Input: part model. Units: mm. Frame: model coordinates. A direction names the side the tool comes from. Coordinates: 2 decimals unless noted, no trailing zeros. Write each loop counter-clockwise with the first axis right and the second up, starting at its lowest first coordinate (ties: lowest second). Pieces come first, ordered by that corner, then holes. Notation, with made-up numbers: M 42.25,15.25 L 49.25,15.25 A34 ccw 49.25,49.25 Z; hole C 50,-24.75 d6. An arc over 180 degrees is marked long. Use one line per item in the form item = value.
Autodesk Inventor part; units mm, degrees
ref_plane "YZ Plane" through (0, 0, 0) normal (1, 0, 0) x (0, 1, 0)
ref_plane "XZ Plane" through (0, 0, 0) normal (0, 1, 0) x (-1, 0, 0)
ref_plane "XY Plane" through (0, 0, 0) normal (0, 0, 1) x (1, 0, 0)
sketch "스케치1" plane through (0, 0, 0) normal (0, 0, 1) x (1, 0, 0)
  line L0 (0, 0) -> (28, 0)
  line L1 (28, 0) -> (28, 33)
  line L2 (28, 33) -> (0, 33)
  line L3 (0, 33) -> (0, 0)
  line L4 (0, 34) -> (28, 34)
  line L5 (28, 34) -> (28, -1)
  line L6 (28, -1) -> (0, -1)
  line L7 (0, -1) -> (0, 34)
  circle A0 centre (-3.95, 14.85) radius 1.65
  circle A1 centre (31.95, 14.85) radius 1.65
  circle A2 centre (14, 14.85) radius 22.1
  line L8 (0, 34) -> (-8.1, 14.85)
  line L9 (-8.1, 14.85) -> (0, -1)
  line L10 (28, -1) -> (36.1, 14.85)
  line L11 (36.1, 14.85) -> (28, 34)
  point P0 (29.3923, 30.7084)
  point P1 (26.609, 33)
  point P2 (1.391, 33)
  point P3 (-1.3923, 30.7084)
  point P4 (0, 31.95)
  point P5 (28, 31.95)
  dimension "d0" = 28
  dimension "d1" = 33
  dimension "d2" = 28
  dimension "d3" = 35
  dimension "d4" = 1
  dimension "d5" = 3.3
  dimension "d6" = 3.3
  dimension "d7" = 35.9
  dimension "d8" = 3.95
  dimension "d9" = 15.85
  dimension "d10" = 44.2
extrude "돌출1" add sketch "스케치1" against normal blind 3.9 contours L3 A2 L2 L1 L0 | L7 L9 L8 A2 L3 | L0 L5 L6 L7 | L1 A2 L11 L10 L5 | A2 L8 L7 L3 | L3 L2 A2 | A2 L2 L1 | L1 L5 L11 A2 | L7 L4 A2 L2 | A2 L4 L2 | L2 A2 L4 L5
extrude "돌출2" add sketch "스케치1" against normal blind 45 contours L3 A2 L2 L1 L0
extrude "돌출3" add sketch "스케치1" along normal blind 2.5 contours L3 A2 L2 L1 L0
properties part number "outlet"
(1) Set-up query: faces 1 (the cylindrical face through (0.7, 32.5, 1.2)), 2 (the cylindrical face through (27.3, 32.5, -24.2)), 3 (the flat face through (14, 33, -24)), 4 (the flat face through (14, 33, 1)). Return all of +Z, -Z, +X, -X, +Y, -Y with unobstructed straight access to the full face (end or side cutting, diameter ignored); none if empty.
Computed:
face_1 = +Z, -X, +Y
face_2 = -Z, +X, +Y
face_3 = -Z, +X, -X, +Y
face_4 = +Z, +X, -X, +Y
(2) Line query: probe 1 along X at (y, z) = (14, -2); probe 2 along X at (y, z) = (24, -8); probe 3 along Y at (x, z) = (-3.95, -2.5). Output: solid intervals per line, ascending.
Computed:
probe_1 = -7.67 to -5.36, -2.54 to 30.54, 33.36 to 35.67
probe_2 = 0 to 28
probe_3 = 6.73 to 13.2, 16.5 to 24.66
(3) Section query D-D on z = -41.5. Return the cut outline in (x, y).
Computed:
outline = M 0,0 L 28,0 L 28,31.95 A22.1 ccw 26.61,33 L 1.39,33 A22.1 ccw 0,31.95 Z
(4) Pull-direction query (X, two-part tool) for faces 5 (the flat face through (0, 16, -24)), 6 (the cylindrical face through (-4.31, 13.24, -1.92)), 7 (the cylindrical face through (30.64, 13.85, -1.92)), 8 (the flat face through (29, 14, 0)); classes: pulls with the +X half, pulls with the -X half, needs draft (parallel to the pull), parting line crosses it, or undercut.
Computed:
face_5 = pulls with the -X half
face_6 = undercut
face_7 = undercut
face_8 = needs draft
(5) Section query B-B on y = 5. Return the cut outline in (x, z).
Computed:
outline = M -3.07,-3.9 L 0,-3.9 L 0,-45 L 28,-45 L 28,-3.9 L 31.07,-3.9 L 31.07,0 L 28,0 L 28,2.5 L 0,2.5 L 0,0 L -3.07,0 Z
(6) Section query C-C on x = 14.5. Return the cut outline in (y, z).
Computed:
outline = M -1,-3.9 L 0,-3.9 L 0,-45 L 33,-45 L 33,-3.9 L 34,-3.9 L 34,0 L 33,0 L 33,2.5 L 0,2.5 L 0,0 L -1,0 Z
(7) Section query A-A on x = 31.95. Return the cut outline in (y, z), plus the area to 3 significant figures.
Computed:
outline = M 6.73,-3.9 L 13.2,-3.9 L 13.2,0 L 6.73,0 Z; M 16.5,-3.9 L 24.66,-3.9 L 24.66,0 L 16.5,0 Z
area = 57.1 mm^2
(8) First-contact query: pin 1 Ø2 at (x, z) = (13, 2) entering from -Y; pin 2 Ø9.5 at (y, z) = (13.5, -30) entering from -X; pin 3 Ø3 at (y, z) = (12.5, 1) entering from -X; pin 4 Ø2.5 at (x, y) = (31.95, 14.85) entering from -Z. Flat tips, straight axial feed; report the tip coordinate or a pass-through.
Computed:
pin_1 = 0
pin_2 = 0
pin_3 = -7.47
pin_4 = through
